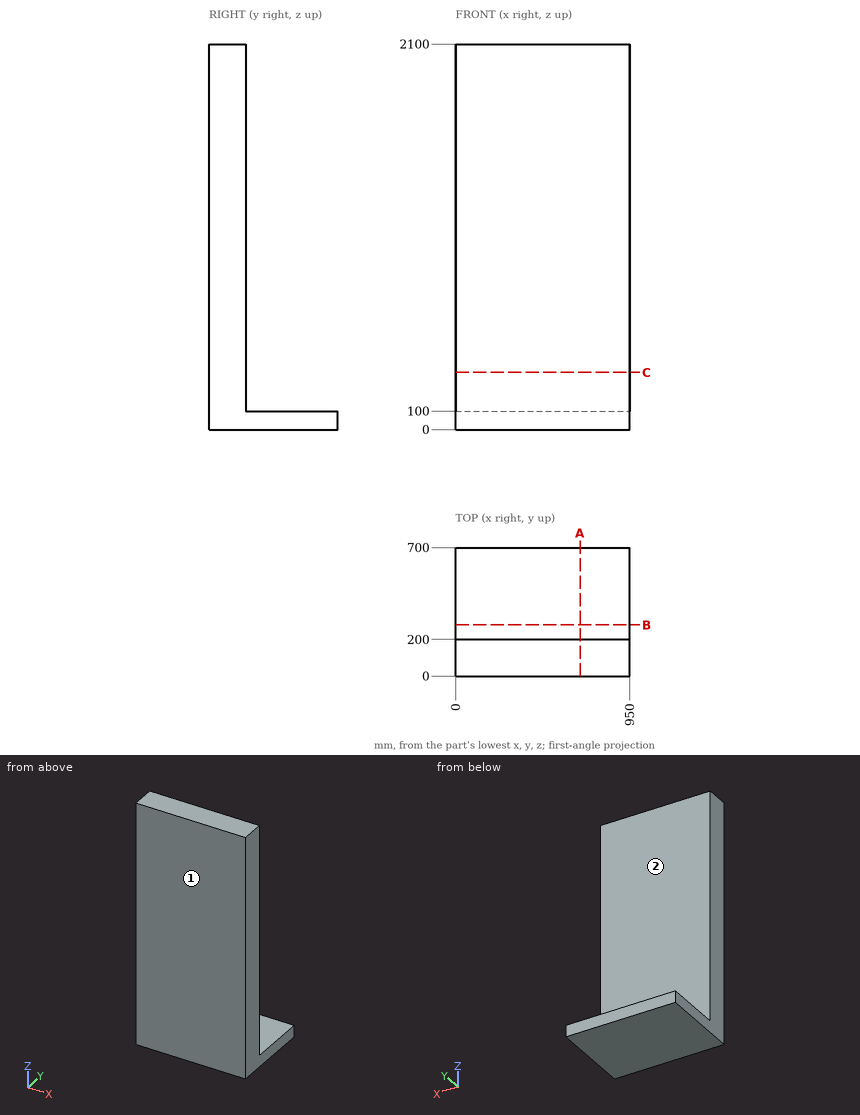
Design review of the part shown in the three views and the two pictorial views. Dimensions are in mm from the part's minimum x, y and z. A direction names the side the tool comes from. Give positions to 0.01 mm unless a question says otherwise; leave off trailing zeros. Write each loop counter-clockwise with the first axis right and the second up, starting at its lowest first coordinate (ties: lowest second). Pieces come first, ordered by that corner, then holes. Notation, with made-up numbers: M -3,48 L 31,48 A23 cw 31,69 Z; hole C 75,9.5 d5. An arc over 180 degrees is marked long. Answer as CSV lines item,"result".
1. Consider section A-A, the plane x = 679. Write out the cut boundary in (y, z), then the cut area to 3 significant figures.
Findings:
outline,"M 0,0 L 700,0 L 700,100 L 200,100 L 200,2100 L 0,2100 Z"
area,"470,000 mm2"
2. For pin 1 (8 mm diameter, centred on x = 372, y = 134.5, fed in from -Z), flat-tipped, find the tip position at first contact; note if it passes through.
Findings:
pin 1,"stops at z = 0"
3. Consider section B-B, the plane y = 279. Write out the cut boundary in (x, z), then the cut area to 3 significant figures.
Findings:
outline,"M 0,0 L 950,0 L 950,100 L 0,100 Z"
area,"95,000 mm2"
4. Consider section C-C, the plane z = 311.5. Write out the cut boundary in (x, y), then the cut area to 3 significant figures.
Findings:
outline,"M 0,0 L 950,0 L 950,200 L 0,200 Z"
area,"190,000 mm2"
5. For the marked faces 1 and 2, list the 3-axis set-ups (+Z, -Z, +X, -X, +Y, -Y) from which the entire face can be reached by the end or side of a thin tool; tool diameter is ignored.
Findings:
face 1,"+Z, -Z, +X, -X, -Y"
face 2,"+Z, +X, -X, +Y"
6. Wall thickness on line 1 (Y direction, x = 485.5, z = 2008.5); line 2 (Z direction, x = 383, y = 531.5): over which ranges is each line inside the solid? List them lowest first.
Findings:
line 1,"y = 0 to 200"
line 2,"z = 0 to 100"
